from build123d import *

# Parameters (mm, degrees)
BOSS_EXTRUDE1_DEPTH     = 2.8
F_1_2_20_TAPPED_HOLE1_D = 11.50874


with BuildPart() as part:
    # Sketch1 → Boss-Extrude1 (new body)
    with BuildSketch(Plane.XY):
        Polygon((0, 8), (-6.92820323, 4), (-6.92820323, -4), (0, -8), (6.92820323, -4), (6.92820323, 4), align=None)
    extrude(amount=BOSS_EXTRUDE1_DEPTH)

    # 1/2-20 Tapped Hole1 (through all)
    with Locations(Plane.XY.offset(2.8)):
        with Locations((0, 0)):
            Hole(F_1_2_20_TAPPED_HOLE1_D / 2)

    # Sketch6 → Cut-Revolve4 (revolve, cut)
    with BuildSketch(Plane(origin=(0, 0, 0), x_dir=(0, 0, -1), z_dir=(1, 0, 0))):
        with BuildLine():
            Line((-3.556750554, -8.169183417), (-3.141854791, -1.510155907))
            Line((-3.141854791, -1.510155907), (-3.012564121, -1.510155907))
            ThreePointArc((-3.012564121, -1.510155907), (-2.693421742, -4.779625328), (-2.04498583, -8))
            ThreePointArc((-2.04498583, -8), (-2.70372151, -8.952660986), (-3.556750554, -8.169183417))
        make_face()
        with BuildLine():
            Line((0.212564121, -1.510155907), (0.341854791, -1.510155907))
            Line((0.341854791, -1.510155907), (0.756750554, -8.169183417))
            ThreePointArc((0.756750554, -8.169183417), (-0.09627849, -8.952660986), (-0.75501417, -8))
            ThreePointArc((-0.75501417, -8), (-0.106578258, -4.779625328), (0.212564121, -1.510155907))
        make_face()
    revolve(axis=Axis((0, 0, 0), (0, 0, 1)), mode=Mode.SUBTRACT)


solid = part.part
Part model, mm, in its own coordinate system. Coordinates: 2 decimals unless noted, no trailing zeros. Write each loop counter-clockwise with the first axis right and the second up, starting at its lowest first coordinate (ties: lowest second). Pieces come first, ordered by that corner, then holes. Notation, with made-up numbers: M 80.5,-35 L 136.5,-35 A24 ccw 136.5,-21 Z; hole C 20,-7.5 d6. An arc over 180 degrees is marked long. Return JSON: item names as keys, results as strings.
1. Saw through at B-B, the plane x = 2.5. Write the cut outline in (y, z).
Determined:
{"outline": "M -6.56,0.52 A32.32 ccw -5.18,0.27 L -5.18,2.53 A32.32 ccw -6.56,2.28 Z; M 5.18,0.27 A32.32 ccw 6.56,0.52 L 6.56,2.28 A32.32 ccw 5.18,2.53 Z"}
2. Saw through at C-C, the plane y = 4.5. Write the cut outline in (x, z), then the cut area to 3 significant figures.
Determined:
{"outline": "M -6.06,0.64 A32.1 ccw -3.59,0.27 L -3.59,2.53 A32.1 ccw -6.06,2.16 Z; M 3.59,0.27 A32.1 ccw 6.06,0.64 L 6.06,2.16 A32.1 ccw 3.59,2.53 Z", "area": "9.52 mm²"}
3. Saw through at A-A, the plane z = 1.4. Write the cut outline in (x, y), then the cut area to 4 significant figures.
Determined:
{"outline": "M -6.93,-4 L 0,-8 L 6.93,-4 L 6.93,4 L 0,8 L -6.93,4 Z; hole C 0,0 d11.51", "area": "62.25 mm²"}
4. Pull direction X, two halves, no side cores. Call faces 1 (the face through (-6.928, 0, 1)), 2 (the face through (0.749, 5.705, 1.384)), 3 (the face through (3.416, -6.028, 1.387)): pulls with the +X half, pulls with the -X half, needs draft (parallel to the pull), parting line crosses it, or undercut.
Determined:
{"face 1": "pulls with the -X half", "face 2": "undercut", "face 3": "pulls with the +X half"}
5. Probe L1, parallel to X at y = 0, z = 1; L2, parallel to X at y = 2, z = 0.6; L3, parallel to Y at x = -5, z = 1.4. List the from-to ranges inside material, lowest first.
Determined:
{"L1": "-6.93 to -5.75, 5.75 to 6.93", "L2": "-6.93 to -5.4, 5.4 to 6.93", "L3": "-5.11 to -2.85, 2.85 to 5.11"}
6. Saw through at D-D, the plane x = -6. Write the cut outline in (y, z), then the cut area to 3 significant figures.
Determined:
{"outline": "M -4.54,0.64 A31.85 ccw 4.54,0.64 L 4.54,2.16 A31.85 ccw -4.54,2.16 Z", "area": "17.8 mm²"}
